```python
from build123d import *

# Parameters (mm, degrees)
SKETCH1_R           = 6.5
BOSS_EXTRUDE1_DEPTH = 5.8
SKETCH2_R           = 4.8
CUT_EXTRUDE1_DEPTH  = 1.5875
SKETCH3_R           = 1
BOSS_EXTRUDE2_DEPTH = 1.5875
SKETCH4_R           = 1.525
BOSS_EXTRUDE3_DEPTH = 3
SKETCH5_R           = 0.85
CUT_EXTRUDE2_DEPTH  = 37.973494724
SKETCH6_R           = 1.1
CUT_EXTRUDE3_DEPTH  = 3
FILLET1_R           = 0.2


with BuildPart() as part:
    # Sketch1 → Boss-Extrude1 (new body)
    with BuildSketch(Plane.XY):
        with Locations((-29.082250471, -1.703826149)):
            Circle(SKETCH1_R)
    extrude(amount=BOSS_EXTRUDE1_DEPTH)

    # Sketch2 → Cut-Extrude1 (cut)
    with BuildSketch(Plane(origin=(0, 0, 0), x_dir=(-1, 0, 0), z_dir=(0, 0, -1))):
        with Locations((29.082250471, -1.703826149)):
            Circle(SKETCH2_R)
    extrude(amount=-CUT_EXTRUDE1_DEPTH, mode=Mode.SUBTRACT)

    # Sketch3 → Boss-Extrude2 (add)
    with BuildSketch(Plane(origin=(0, 0, 1.5875), x_dir=(-1, 0, 0), z_dir=(0, 0, -1))):
        with Locations((29.082250471, -1.703826149)):
            Circle(SKETCH3_R)
    extrude(amount=BOSS_EXTRUDE2_DEPTH)

    # Sketch4 → Boss-Extrude3 (add)
    with BuildSketch(Plane(origin=(0, 0, 0), x_dir=(-1, 0, 0), z_dir=(0, 0, -1))):
        with Locations((29.082250471, -1.703826149)):
            Circle(SKETCH4_R)
    extrude(amount=-BOSS_EXTRUDE3_DEPTH)

    # Sketch5 → Cut-Extrude2 (cut, through all)
    with BuildSketch(Plane(origin=(0, 0, 0), x_dir=(-1, 0, 0), z_dir=(0, 0, -1))):
        with Locations((29.082250471, -1.703826149)):
            Circle(SKETCH5_R)
    extrude(amount=-CUT_EXTRUDE2_DEPTH, mode=Mode.SUBTRACT)

    # Sketch6 → Cut-Extrude3 (cut)
    with BuildSketch(Plane.XY.offset(5.8)):
        with Locations((-29.082250471, -1.703826149)):
            Circle(SKETCH6_R)
    extrude(amount=-CUT_EXTRUDE3_DEPTH, mode=Mode.SUBTRACT)

    # Fillet1
    fillet1_edges = [part.edges().sort_by_distance(p)[0] for p in [
        (-27.557250471, -1.703826149, 0),
    ]]
    fillet(fillet1_edges, radius=FILLET1_R)


solid = part.part
```
Read the model definition and answer for the solid it produces. Units are mm, in the model's axes. A direction names the side the tool comes from. Coordinates: 2 decimals unless noted, no trailing zeros. Loops run counter-clockwise (first coordinate to the right, second up) from the corner with the lowest first, then second, coordinate; pieces in that order, holes last. Notation, with made-up numbers: (23, 18) -> (63, 18) arc R28 ccw to (63, 54) -> close; hole circle Ø9 at (72.5, 9.5). An arc over 180 degrees is marked (long way). Return JSON: item names as keys, results as strings.
Item 1: Find section C-C (z = 0.6). Determine the outline of the cut face in (x, y) (3 decimals).
Answers:
{"outline": "circle Ø13 at (-29.082, -1.704); circle Ø3.05 at (-29.082, -1.704); hole circle Ø9.6 at (-29.082, -1.704); hole circle Ø1.7 at (-29.082, -1.704)"}
Item 2: For faces 1 (the cylindrical face through (-29.893, -1.449, 1.38)), 2 (the cylindrical face through (-24.287, -1.493, 0.783)), determine the directions among +Z, -Z, +X, -X, +Y, -Y from which every point of the face is accessible in a straight line to the end or side of a thin tool.
Answers:
{"face 1": "+Z, -Z", "face 2": "-Z"}
Item 3: Find the intervals of material crossed by probe 1 along Z at (x, y) = (-32, 0.5); probe 2 along X at (y, z) = (-1.25, 5); probe 3 along X at (y, z) = (-4.75, 0.65), in increasing order.
Answers:
{"probe 1": "z = 1.59 to 5.8", "probe 2": "x = -35.57 to -30.08, -28.08 to -22.6", "probe 3": "x = -34.82 to -32.79, -25.37 to -23.34"}
Item 4: For a pull along X with two mould halves and no side action, classify faces 3 (the cylindrical face through (-28.07, -2.13, 4.32)), 4 (the flat face through (-27.7, -1.6, 5.8)), 5 (the cylindrical face through (-22.882, 0.249, 2.859)), 6 (the flat face through (-31, -2, 1.588)) as +X half, -X half, draft (parallel to the pull), parting line (faces both ways), or undercut.
Answers:
{"face 3": "undercut", "face 4": "draft", "face 5": "parting line", "face 6": "undercut"}
Item 5: Find section B-B (y = 2.25). Determine the outline of the cut face in (x, z), plus the area to 3 significant figures.
Answers:
{"outline": "(-34.24, 0) -> (-31.8, 0) -> (-31.8, 1.59) -> (-26.36, 1.59) -> (-26.36, 0) -> (-23.92, 0) -> (-23.92, 5.8) -> (-34.24, 5.8) -> close", "area": "51.2 mm2"}
Item 6: Find section D-D (z = 5.05). Determine the outline of the cut face in (x, y), plus the area to 3 significant figures.
Answers:
{"outline": "circle Ø13 at (-29.08, -1.7); hole circle Ø2.2 at (-29.08, -1.7)", "area": "129 mm2"}
Item 7: Find section A-A (x = -25.5). Determine the outline of the cut face in (y, z), plus the area to 3 significant figures.
Answers:
{"outline": "(-7.13, 0) -> (-4.9, 0) -> (-4.9, 1.59) -> (1.49, 1.59) -> (1.49, 0) -> (3.72, 0) -> (3.72, 5.8) -> (-7.13, 5.8) -> close", "area": "52.8 mm2"}
Item 8: A flat-ended cylindrical pin translates along its axis: P1, Ø1, axis at x = -33, z = 1, coming from the +Y side. Find the tip coordinate at first contact, or state that the pin passes through.
Answers:
{"P1": "stops at y = 3.83"}
